from build123d import *

# Parameters (mm, degrees)
F0_R            = 31.75
F1_DEPTH        = 304.8
F2_R            = 28.575
F3_DEPTH        = 292.1
F4_R            = 57.15
F4_R_2          = 31.75
F5_DEPTH        = 12.7
F7_DEPTH        = 3.175
F7_COPIES_COUNT = 4
F8_R            = 31.75
F9_DEPTH        = 50.8
F10_R           = 29.21
F11_DEPTH       = 87.884


# Not quite as in the source:
# - a pattern or mirror of a feature is missing from the dataset's text; its kind, count and spacing are read off the source's solid


with BuildPart() as f1:
    # F0 (on Top) → F1 (new body)
    with BuildSketch(Plane.XY):
        Circle(F0_R)
    extrude(amount=F1_DEPTH)

    # F2 (on face) → F3 (cut)
    with BuildSketch(Plane.XY.offset(304.8)):
        Circle(F2_R)
    extrude(amount=-F3_DEPTH, mode=Mode.SUBTRACT)

    # F4 (on face) → F5 (join)
    with BuildSketch(Plane.XY.offset(304.8)):
        Circle(F4_R)
        Circle(F4_R_2, mode=Mode.SUBTRACT)
    extrude(amount=-F5_DEPTH)

    # F6 (on Right) → F7 (join, symmetric)
    with BuildSketch(Plane.YZ):
        Polygon((30.9059452266, 236.7404699326), (56.9043979049, 292.3926711082), (30.9059452266, 290.2498841286), align=None)
    f7 = extrude(amount=F7_DEPTH, both=True)

    # F7_copies: F7 ×4 about axis
    f7_copies_axis = Axis((0, 0, 0), (0, 0, 1))
    for i in range(1, F7_COPIES_COUNT):
        add(f7.rotate(f7_copies_axis, i * 360 / F7_COPIES_COUNT))

    # F8 (on face) → F9 (join)
    with BuildSketch(Plane.XY.offset(304.8)):
        Circle(F8_R)
    extrude(amount=F9_DEPTH)

    # F10 (on face) → F11 (cut)
    with BuildSketch(Plane.XY.offset(355.6)):
        Circle(F10_R)
    extrude(amount=-F11_DEPTH, mode=Mode.SUBTRACT)


solid = f1.part
Work out the finished part from the listing and answer in its coordinate system (mm). A direction names the side the tool comes from. Coordinates: 2 decimals unless noted, no trailing zeros. Write each loop counter-clockwise with the first axis right and the second up, starting at its lowest first coordinate (ties: lowest second). Pieces come first, ordered by that corner, then holes. Notation, with made-up numbers: M -5.75,-9 L 33.25,-9 A27 ccw 33.25,18 Z; hole C 14.25,-18 d5. An arc over 180 degrees is marked long. Use one line per item in the form item = value. Start each with the question number.
1. A tool of negligible diameter and unlimited length cuts with its end or side. For faces 1 (the face through (-41, 3.175, 272)), 2 (the face through (-41, -3.175, 272)), 3 (the face through (41, -3.175, 272)), 4 (the face through (-6.883, -30.995, 329.844)), from which of +Z, -Z, +X, -X, +Y, -Y can it reach the whole face along a straight path? Write none if from no direction.
2. The mould has two halves that part along Y. Classify faces 5 (the face through (3.175, -41, 272)), 6 (the face through (-21.53, 19.74, 312.27)), 7 (the face through (-57.095, 2.513, 298.539)): released by +Y, released by -Y, zero draft, split by the parting line, or undercut.
3. The part is cut by section D-D (y = 49.5). Give the vertices of the cut face in (x, z) (3 decimals), plus the area to 3 significant figures.
4. The part is cut by section C-C (x = 46.5). Give the vertices of the cut face in (y, z) (3 decimals), plus the area to 3 significant figures.
5. Straight lines are drawn through the part: probe 1 along Y at (x, z) = (0, 84.5) (3 decimals); probe 2 along Z at (x, y) = (37, -21.5); probe 3 along Y at (x, z) = (13, 229.5). For each, find the intervals that lie inside material, in ascending order. Write a range as from..to.
6. Each of these flat-tipped pins is pushed along its axis until it touches: P1, Ø1, axis at y = -22, z = 120.5, coming from the -X side; P2, Ø12, axis at y = -7.5, z = 105.5, coming from the +X side; P3, Ø12.5, axis at x = 46.5, z = 267, coming from the -Y side (3 decimals). Where does it stop, or does it pass through?
7. The part is cut by section B-B (y = 0). Give the vertices of the cut face in (x, z) (3 decimals), plus the area to 3 significant figures.
8. The part is cut by section A-A (z = 248.5). Give the vertices of the cut face in (x, y) (3 decimals), plus the area to 3 significant figures.
Evaluation:
q1.face_1 = -Z, -X, +Y
q1.face_2 = -Z, -X, -Y
q1.face_3 = -Z, +X, -Y
q1.face_4 = +Z
q2.face_5 = zero draft
q2.face_6 = undercut
q2.face_7 = split by the parting line
q3.outline = M -28.563,292.1 L 28.563,292.1 L 28.563,304.8 L -28.563,304.8 Z; M -3.175,276.543 L 3.175,276.543 L 3.175,291.782 L -3.175,291.782 Z
q3.area = 822 mm^2
q4.outline = M -33.225,292.1 L 33.225,292.1 L 33.225,304.8 L -33.225,304.8 Z; M -3.175,270.121 L 3.175,270.121 L 3.175,291.535 L -3.175,291.535 Z
q4.area = 980 mm^2
q5.probe_1 = -31.75..-28.575, 28.575..31.75
q5.probe_2 = 292.1..304.8
q5.probe_3 = -28.97..-25.45, 25.45..28.97
q6.P1 = -23.36
q6.P2 = 31.71
q6.P3 = -3.175
q7.outline = M -57.15,292.1 L -56.768,292.1 L -31.75,238.547 L -31.75,0 L 31.75,0 L 31.75,238.547 L 56.768,292.1 L 57.15,292.1 L 57.15,304.8 L 31.75,304.8 L 31.75,355.6 L 29.21,355.6 L 29.21,267.716 L 28.575,267.716 L 28.575,12.7 L -28.575,12.7 L -28.575,267.716 L -29.21,267.716 L -29.21,355.6 L -31.75,355.6 L -31.75,304.8 L -57.15,304.8 Z; hole M -53.353,292.1 L -31.75,290.319 L -31.75,292.1 Z; hole M 31.75,290.319 L 53.353,292.1 L 31.75,292.1 Z
q7.area = 4,820 mm^2
q8.outline = M -36.4,-3.175 L -31.591,-3.175 A31.75 ccw -3.175,-31.591 L -3.175,-36.4 L 3.175,-36.4 L 3.175,-31.591 A31.75 ccw 31.591,-3.175 L 36.4,-3.175 L 36.4,3.175 L 31.591,3.175 A31.75 ccw 3.175,31.591 L 3.175,36.4 L -3.175,36.4 L -3.175,31.591 A31.75 ccw -31.591,3.175 L -36.4,3.175 Z; hole C 0,0 d57.15
q8.area = 721 mm^2
